from build123d import *

# Parameters (mm, degrees)
BOSS_EXTRUDE2_DEPTH = 6.35
FILLET1_R           = 6.35
SKETCH2_R           = 2.4892
CUT_EXTRUDE1_DEPTH  = 204.913109234


with BuildPart() as part:
    # Sketch1 → Boss-Extrude2 (new body)
    with BuildSketch(Plane.XY):
        Polygon((51.914761179, 0), (77.314761179, 0), (77.314761179, -101.6), (-141.760238821, -101.6), (-141.760238821, -76.2), (-176.685238821, -76.2), (-176.685238821, 0), (-151.285238821, 0), (-151.285238821, -50.8), (-132.235238821, -50.8), (-132.235238821, -82.55), (51.914761179, -82.55), align=None)
        with BuildLine():
            Line((-87.785238821, -88.9), (-11.585238821, -88.9))
            ThreePointArc((-11.585238821, -88.9), (-8.410238821, -92.075), (-11.585238821, -95.25))
            Line((-11.585238821, -95.25), (-87.785238821, -95.25))
            ThreePointArc((-87.785238821, -95.25), (-90.960238821, -92.075), (-87.785238821, -88.9))
        make_face(mode=Mode.SUBTRACT)
    extrude(amount=BOSS_EXTRUDE2_DEPTH)

    # Fillet1
    fillet1_edges = [part.edges().sort_by_distance(p)[0] for p in [
        (-176.685238821, 0, 3.175),
        (-151.285238821, 0, 3.175),
        (-151.285238821, -50.8, 3.175),
        (-132.235238821, -50.8, 3.175),
        (-132.235238821, -82.55, 3.175),
        (51.914761179, -82.55, 3.175),
        (51.914761179, 0, 3.175),
        (77.314761179, 0, 3.175),
        (77.314761179, -101.6, 3.175),
        (-141.760238821, -101.6, 3.175),
        (-141.760238821, -76.2, 3.175),
        (-176.685238821, -76.2, 3.175),
    ]]
    fillet(fillet1_edges, radius=FILLET1_R)

    # Sketch2 → Cut-Extrude1 (cut, through all)
    with BuildSketch(Plane.XY.offset(6.35)):
        with Locations((64.614761179, -6.35)):
            Circle(SKETCH2_R)
        with Locations((64.614761179, -31.75)):
            Circle(SKETCH2_R)
        with Locations((64.614761179, -57.15)):
            Circle(SKETCH2_R)
        with Locations((-163.985238821, -6.35)):
            Circle(SKETCH2_R)
        with Locations((-163.985238821, -31.75)):
            Circle(SKETCH2_R)
        with Locations((-163.985238821, -57.15)):
            Circle(SKETCH2_R)
    extrude(amount=-CUT_EXTRUDE1_DEPTH, mode=Mode.SUBTRACT)


solid = part.part
The listing builds one solid part. Answer for the finished solid, in the listing's coordinates (mm). A direction names the side the tool comes from. Coordinates: 2 decimals unless noted, no trailing zeros. Write each loop counter-clockwise with the first axis right and the second up, starting at its lowest first coordinate (ties: lowest second). Pieces come first, ordered by that corner, then holes. Notation, with made-up numbers: (77.5, 11) - (104.5, 11) arc R24 ccw to (104.5, 37) - close; hole circle Ø7 at (40.5, 77). An arc over 180 degrees is marked (long way). Put each result on its own line as item: value.
1. Find the intervals of material crossed by line 1 along X through (y, z) = (-25, 5); line 2 along Y through (x, z) = (-66, 5.75); line 3 along X through (y, z) = (-86.5, 1.5), in increasing order. Write a range as from..to.
Answer sheet:
line 1: x = -176.69..-151.29, 51.91..77.31
line 2: y = -101.6..-95.25, -88.9..-82.55
line 3: x = -141.76..77.31
2. The part is cut by section A-A on x = -48. Give the vertices of the cut face in (y, z), plus the area to 3 significant figures.
Answer sheet:
outline: (-101.6, 0) - (-95.25, 0) - (-95.25, 6.35) - (-101.6, 6.35) - close; (-88.9, 0) - (-82.55, 0) - (-82.55, 6.35) - (-88.9, 6.35) - close
area: 80.6 mm^2
3. The part is cut by section B-B on y = -27. Give the vertices of the cut face in (x, z).
Answer sheet:
outline: (-176.69, 0) - (-151.29, 0) - (-151.29, 6.35) - (-176.69, 6.35) - close; (51.91, 0) - (77.31, 0) - (77.31, 6.35) - (51.91, 6.35) - close
4. The part is cut by section D-D on x = 5. Give the vertices of the cut face in (y, z), plus the area to 3 significant figures.
Answer sheet:
outline: (-101.6, 0) - (-82.55, 0) - (-82.55, 6.35) - (-101.6, 6.35) - close
area: 121 mm^2
5. Flat-ended cylindrical pins translate along their axes: pin 1 Ø3 at (y, z) = (-89.5, 3) entering from -X; pin 2 Ø3 at (x, y) = (64.61, -57.15) entering from -Z; pin 3 Ø1.9 at (x, z) = (-160.5, 3) entering from -Y; pin 4 Ø8 at (x, y) = (64.61, -6.35) entering from +Z. Find the tip coordinate at first contact, or state that the pin passes through.
Answer sheet:
pin 1: stops at x = -141.76
pin 2: passes through
pin 3: stops at y = -76.2
pin 4: stops at z = 6.35
6. A tool of negligible diameter and unlimited length cuts with its end or side. For faces 4 (the face through (65, 0, 3)), 5 (the face through (-132.235, -67, 3)), 6 (the face through (-8.41, -92.01, 3.13)), from which of +Z, -Z, +X, -X, +Y, -Y can it reach the whole face along a straight path? Write none if from no direction.
Answer sheet:
face 4: +Z, -Z, +X, -X, +Y
face 5: +Z, -Z, +Y
face 6: +Z, -Z
7. Determine the mould class of faces 1 (the face through (-159, -76.2, 3)), 2 (the face through (-143.57, -78.11, 3.22)), 3 (the face through (-130.326, -80.739, 3.219)) for opening direction X: pulls with the +X half, pulls with the -X half, needs draft (parallel to the pull), parting line crosses it, or undercut.
Answer sheet:
face 1: needs draft
face 2: pulls with the -X half
face 3: undercut
8. The part is cut by section C-C on z = 1. State how many separate pieces and enclosed holes the cut face has, plus the area to 3 significant figures.
Answer sheet:
separate pieces: 1
enclosed holes: 7
area: 8,080 mm^2
